Could you check a few things on this drawing? It's one solid part, dimensions in mm from its lowest x, y, z. A direction names the side the tool comes from. Coordinates: 2 decimals unless noted, no trailing zeros. Order: outer loops, then holes, each group sorted by start corner. A loop starts at its lowest first (then second) coordinate and runs counter-clockwise, first axis right, second up. Notation, with made-up numbers: (-25.75, 3) -> (10.25, 3) arc R24 ccw to (10.25, 33) -> close; hole circle Ø10 at (54, 47.25). An arc over 180 degrees is marked (long way). Answer as CSV lines item,"result".
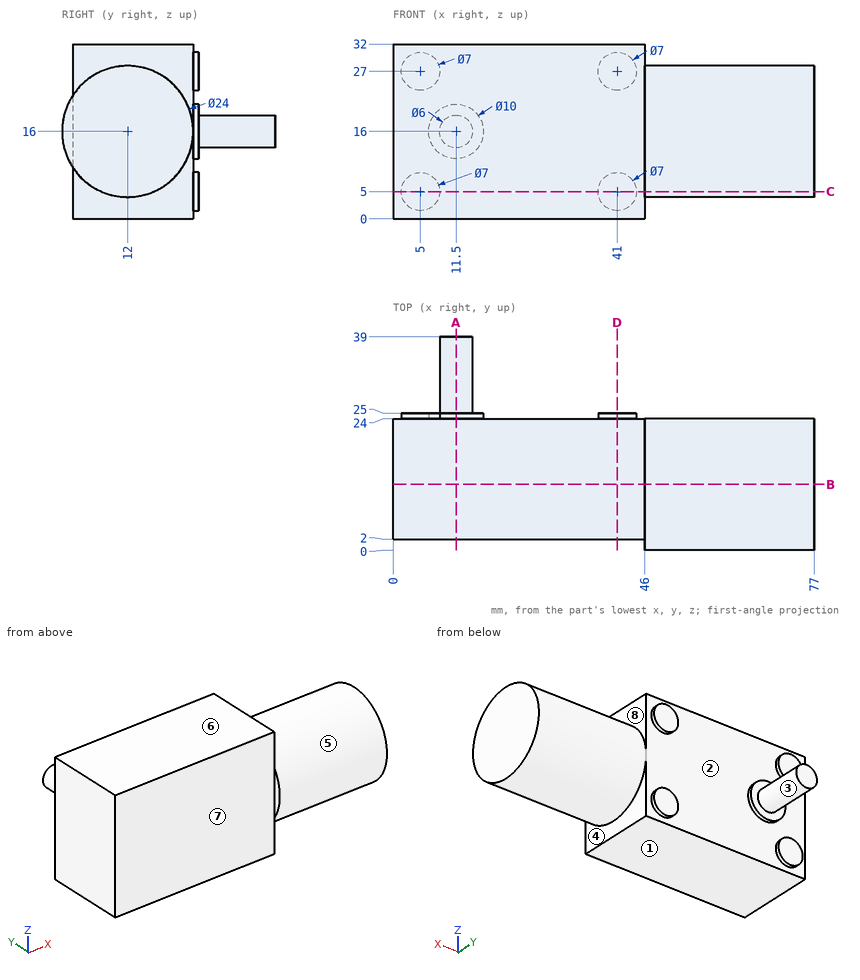
Q1. Imagine slicing it at C-C (z = 5). List the corners of the cut face in (x, y) for me.
Solution:
outline,"(0, 2) -> (46, 2) -> (46, 7.2) -> (77, 7.2) -> (77, 16.8) -> (46, 16.8) -> (46, 24) -> (44.5, 24) -> (44.5, 25) -> (37.5, 25) -> (37.5, 24) -> (8.5, 24) -> (8.5, 25) -> (1.5, 25) -> (1.5, 24) -> (0, 24) -> close"
Q2. If I drill on line 1 (Y direction, x = 42, z = 7); line 2 (Y direction, x = 14, z = 28.5); line 3 (Z direction, x = 60.5, y = 16.5), over which ranges is the centre line in solid material (lowest first)?
Solution:
line 1,"2 to 25"
line 2,"2 to 24"
line 3,"4.88 to 27.12"
Q3. For P1, Ø2, axis at y = 25.5, z = 24, coming from the +X side; P2, Ø1.5, axis at y = 29, z = 13.5, coming from the +X side; P3, Ø6, axis at x = 39.5, y = 13, coming from the -Z side; P4, Ø5.5, axis at x = 3.5, z = 6.5, coming from the +Y side, each with a flat end and sliding along its axis, tell me the tip position at first contact or that it passes through.
Solution:
P1,"x = 43.77"
P2,"x = 13.94"
P3,"z = 0"
P4,"y = 25"
Q4. Imagine slicing it at D-D (x = 41). List the corners of the cut face in (y, z) for me, and give its area (3 significant figures).
Solution:
outline,"(2, 0) -> (24, 0) -> (24, 1.5) -> (25, 1.5) -> (25, 8.5) -> (24, 8.5) -> (24, 23.5) -> (25, 23.5) -> (25, 30.5) -> (24, 30.5) -> (24, 32) -> (2, 32) -> close"
area,"718 mm2"
Q5. Which directions (+Z, -Z, +X, -X, +Y, -Y) give clear straight access to the entire face, cutting with the end or side of a thin tool? Please do the marked faces 5, 6, 7 and 8.
Solution:
face 5,"+X"
face 6,"+Z, +X, -X, +Y, -Y"
face 7,"+Z, -Z, -X, -Y"
face 8,"+Z, +X"
Q6. We'd pull the mould along Z, two halves only. Please class the marked faces 1, 2, 3 and 4: pulls with the +Z half, pulls with the -Z half, needs draft (parallel to the pull), parting line crosses it, or undercut.
Solution:
face 1,"pulls with the -Z half"
face 2,"undercut"
face 3,"parting line crosses it"
face 4,"needs draft"
Q7. Imagine slicing it at A-A (x = 11.5). List the corners of the cut face in (y, z) for me.
Solution:
outline,"(2, 0) -> (24, 0) -> (24, 11) -> (25, 11) -> (25, 13) -> (39, 13) -> (39, 19) -> (25, 19) -> (25, 21) -> (24, 21) -> (24, 32) -> (2, 32) -> close"
Q8. Imagine slicing it at B-B (y = 12). List the corners of the cut face in (x, z) for me.
Solution:
outline,"(0, 0) -> (46, 0) -> (46, 4) -> (77, 4) -> (77, 28) -> (46, 28) -> (46, 32) -> (0, 32) -> close"
